The model under review builds one solid part; all positions refer to its coordinate system, in mm. Face numbers are marked on the shaded views. Give positions to 0.01 mm unless a question says otherwise; leave off trailing zeros. Order: outer loops, then holes, each group sorted by start corner. A loop starts at its lowest first (then second) coordinate and runs counter-clockwise, first axis right, second up. Notation, with made-up numbers: (-13.5, 20) - (37.5, 20) arc R19 ccw to (37.5, 31) - close; hole circle Ø9 at (20, -26). An arc over 180 degrees is marked (long way). Put each result on its own line as item: value.
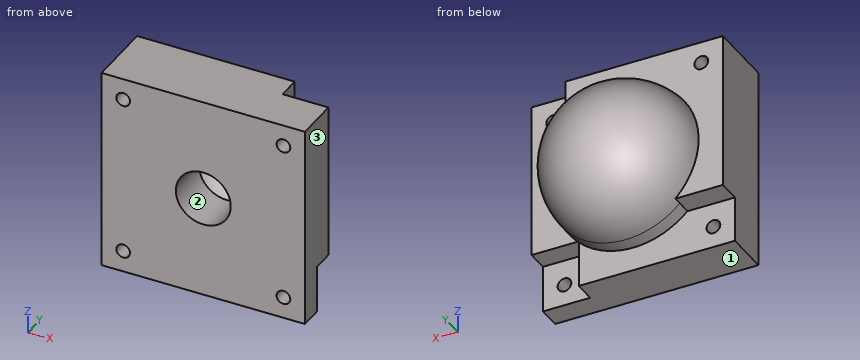
```python
from build123d import *

# Parameters (mm, degrees)
SKETCH3_W               = 44.4
SKETCH3_H               = 44.4
BOSS_EXTRUDE1_DEPTH     = 9.7
SKETCH5_R               = 6
CUT_EXTRUDE2_DEPTH      = 14.3
BOSS_EXTRUDE2_DEPTH     = 5
CUT_EXTRUDE3_DEPTH      = 35.870626966
CUT_EXTRUDE3_DEPTH_BACK = 35.870626966
SKETCH7_R               = 1.5
SKETCH8_W               = 10.3
SKETCH8_H               = 10.3
CUT_EXTRUDE4_DEPTH      = 4.7


with BuildPart() as part:
    # Sketch2 → Revolve1 (revolve)
    with BuildSketch(Plane.XY, mode=Mode.PRIVATE) as revolve1_sk:
        with BuildLine():
            Line((-10, 0), (-12, 0))
            ThreePointArc((-12, 0), (-8.485281374, 8.485281374), (0, 12))
            Line((0, 12), (0, 17))
            ThreePointArc((0, 17), (-12.02081528, 12.02081528), (-17, 0))
            Line((-17, 0), (-17, -3.175))
            Line((-17, -3.175), (-10, -3.175))
            Line((-10, -3.175), (-10, 0))
        make_face()
    revolve(revolve1_sk.sketch.rotate(Axis((0, 12, 0), (0, 1, 0)), 180), axis=Axis((0, 12, 0), (0, 1, 0)))

    # Sketch3 → Boss-Extrude1 (add)
    with BuildSketch(Plane.XZ.offset(3.175)):
        Rectangle(SKETCH3_W, SKETCH3_H)
    extrude(amount=BOSS_EXTRUDE1_DEPTH)

    # Sketch5 → Cut-Extrude2 (cut)
    with BuildSketch(Plane.XZ.offset(12.875)):
        Circle(SKETCH5_R)
    extrude(amount=-CUT_EXTRUDE2_DEPTH, mode=Mode.SUBTRACT)

    # Sketch6 → Boss-Extrude2 (add)
    with BuildSketch(Plane(origin=(0, -3.175, 0), x_dir=(1, 0, 0), z_dir=(0, 1, 0))):
        with BuildLine():
            Line((-22.2, -22.2), (-22.2, 12.2))
            Line((-22.2, 12.2), (-11.83, 12.2))
            ThreePointArc((-11.83, 12.2), (-11.83, -11.83), (12.2, -11.83))
            Line((12.2, -11.83), (12.2, -22.2))
            Line((12.2, -22.2), (-22.2, -22.2))
        make_face()
    extrude(amount=BOSS_EXTRUDE2_DEPTH)

    # Sketch7 → Cut-Extrude3 (cut, two sides: drawn at the far end of the back side and taken through both)
    with BuildSketch(Plane(origin=(0, 1.825, 0), x_dir=(1, 0, 0), z_dir=(0, 1, 0)).offset(-CUT_EXTRUDE3_DEPTH_BACK)):
        with Locations(Location((-17.5, -17.5, 0), (0, 0, 180))):
            Circle(SKETCH7_R)
        with Locations(Location((17.5, -17.5, 0), (0, 0, 180))):
            Circle(SKETCH7_R)
        with Locations(Location((17.5, 17.5, 0), (0, 0, 180))):
            Circle(SKETCH7_R)
        with Locations(Location((-17.5, 17.5, 0), (0, 0, 180))):
            Circle(SKETCH7_R)
    extrude(amount=CUT_EXTRUDE3_DEPTH + CUT_EXTRUDE3_DEPTH_BACK, mode=Mode.SUBTRACT)

    # Sketch8 → Cut-Extrude4 (cut)
    with BuildSketch(Plane(origin=(0, -3.175, 0), x_dir=(1, 0, 0), z_dir=(0, 1, 0))):
        with Locations((17.05, 17.05)):
            Rectangle(SKETCH8_W, SKETCH8_H)
    extrude(amount=-CUT_EXTRUDE4_DEPTH, mode=Mode.SUBTRACT)


solid = part.part
```
(1) Clearance check with flat-ended pins moving along their axes: pin 1 Ø4 at (x, y) = (19, -5) entering from -Z; pin 2 Ø5 at (x, z) = (17.5, -17.5) entering from -Y (3 decimals); pin 3 Ø1.5 at (x, z) = (-0.5, -10) entering from +Y; pin 4 Ø8 at (x, y) = (-10.5, 7) entering from +Z. State where each tip first meets the part, or that it passes through.
The answers:
pin 1: z = -11.9
pin 2: y = -12.875
pin 3: y = 14.26
pin 4: z = 14.65
(2) Wall thickness on L1, parallel to Z at x = 17.5, y = -9.9; L2, parallel to Z at x = 17.5, y = -7.25; L3, parallel to Y at x = 3, z = 19 (3 decimals): over which ranges is each line inside the solid? List them lowest first.
The answers:
L1: -22.2 to -19, -16 to 16, 19 to 22.2
L2: -11.9 to 16, 19 to 22.2
L3: -12.875 to 1.825
(3) Take a section at D-D, the plane y = -9.5. Write out the cut boundary in (x, z), then the cut area to 3 significant figures.
The answers:
outline: (-22.2, -22.2) - (22.2, -22.2) - (22.2, 22.2) - (-22.2, 22.2) - close; hole circle Ø3 at (-17.5, -17.5); hole circle Ø3 at (-17.5, 17.5); hole circle Ø12 at (0, 0); hole circle Ø3 at (17.5, -17.5); hole circle Ø3 at (17.5, 17.5)
area: 1,830 mm^2
(4) Take a section at C-C, the plane y = -6. Write out the cut boundary in (x, z).
The answers:
outline: (-22.2, -22.2) - (11.9, -22.2) - (11.9, -11.9) - (22.2, -11.9) - (22.2, 22.2) - (-22.2, 22.2) - close; hole circle Ø3 at (-17.5, -17.5); hole circle Ø3 at (-17.5, 17.5); hole circle Ø12 at (0, 0); hole circle Ø3 at (17.5, 17.5)
(5) Take a section at A-A, the plane x = -17.5. Write out the cut boundary in (y, z) (3 decimals).
The answers:
outline: (-12.875, -22.2) - (-3.175, -22.2) - (-3.175, -19) - (-12.875, -19) - close; (-12.875, -16) - (-3.175, -16) - (-3.175, -12.2) - (1.825, -12.2) - (1.825, 16) - (-12.875, 16) - close; (-12.875, 19) - (1.825, 19) - (1.825, 22.2) - (-12.875, 22.2) - close
(6) The part is to be moulded in two halves that separate along Z. For the marked faces 1, 2 and 3, say which applies: pulls with the +Z half, pulls with the -Z half, needs draft (parallel to the pull), parting line crosses it, or undercut.
The answers:
face 1: pulls with the -Z half
face 2: undercut
face 3: needs draft
(7) Take a section at B-B, the plane z = 17.5. Write out the cut boundary in (x, y) (3 decimals).
The answers:
outline: (-22.2, -12.875) - (-19, -12.875) - (-19, 1.825) - (-22.2, 1.825) - close; (-16, -12.875) - (16, -12.875) - (16, -3.175) - (12.2, -3.175) - (12.2, 1.825) - (-16, 1.825) - close; (19, -12.875) - (22.2, -12.875) - (22.2, -3.175) - (19, -3.175) - close
